Geometry: final body of the model. Coordinates: model frame, mm. Give positions to 0.01 mm unless a question says otherwise; leave off trailing zeros. Write each loop counter-clockwise with the first axis right and the second up, starting at its lowest first coordinate (ties: lowest second). Pieces come first, ordered by that corner, then holes.
Q1. Section B-B (x = 0). Return the cut outline in (y, z), plus the area to 3 significant figures.
Q2. Section D-D (y = -42). Return the cut outline in (x, z), plus the area to 3 significant figures.
Q3. Pin query (flat end, axial travel): pin 1 Ø1 at (y, z) = (-44, -9.5) entering from +X; pin 2 Ø8 at (x, y) = (-6.5, -110) entering from +Z; pin 3 Ø10 at (x, y) = (-4, -24) entering from -Z; pin 4 Ø10 at (x, y) = (8.5, -47) entering from -Z. Return the tip coordinate at first contact, or that it passes through.
Q4. Section C-C (y = -130). Return the cut outline in (x, z).
Q5. Mould query, pull axis Z, two halves, no side actions, for faces 1 (the cylindrical face through (-1.73, -68.53, -7.81)), 2 (the cylindrical face through (-0.113, -127.615, 0.751)), 3 (the flat face through (2, 0, -8)). Classes: +Z half, -Z half, draft (parallel to the pull), parting line (faces both ways), or undercut.
Q6. Line query: line 1 (Z direction, x = 0.5, y = -130); line 2 (Y direction, x = -3.25, z = 0); line 3 (Z direction, x = -4.5, y = -130). Output: solid intervals per line, ascending.
Q7. Section A-A (z = 0). Return the cut outline in (x, y), plus the area to 3 significant figures.
from build123d import *

# Parameters (mm, degrees)
F0_R     = 8
F1_DEPTH = 140
F0_R_2   = 12
F2_DEPTH = 5
F3_SIZE  = 1
F5_R     = 2.5
F6_DEPTH = 20.001


with BuildPart() as f1:
    # F0 (on Front) → F1 (new body)
    with BuildSketch(Plane.XZ):
        Circle(F0_R)
    extrude(amount=F1_DEPTH)

    # F0 (on Front) → F2 (join)
    with BuildSketch(Plane.XZ):
        Circle(F0_R_2)
        Circle(F0_R, mode=Mode.SUBTRACT)
        Circle(F0_R)
    extrude(amount=-F2_DEPTH)

    # F3
    f3_edges = [f1.edges().sort_by_distance(p)[0] for p in [
        (-12, 5, 0),
        (-8, -140, 0),
    ]]
    chamfer(f3_edges, length=F3_SIZE)

    # F5 (on offset) → F6 (cut, through all)
    with BuildSketch(Plane.YZ.offset(-8)):
        with Locations((-130, 0)):
            Circle(F5_R)
    extrude(amount=F6_DEPTH, mode=Mode.SUBTRACT)


solid = f1.part
Computed:
1. outline: (-140, -7) - (-139, -8) - (0, -8) - (0, -12) - (4, -12) - (5, -11) - (5, 11) - (4, 12) - (0, 12) - (0, 8) - (-139, 8) - (-140, 7) - close; hole circle Ø5 at (-130, 0)
1. area: 2,340 mm2
2. outline: circle Ø16 at (0, 0)
2. area: 201 mm2
3. pin 1: passes through
3. pin 2: stops at z = 7.6
3. pin 3: stops at z = -8
3. pin 4: stops at z = -7.19
4. outline: (-7.6, -2.5) arc R8 ccw to (7.6, -2.5) - close; (-7.6, 2.5) - (7.6, 2.5) arc R8 ccw to start
5. face 1: parting line
5. face 2: undercut
5. face 3: draft
6. line 1: z = -7.98 to -2.5, 2.5 to 7.98
6. line 2: y = -140 to -132.5, -127.5 to 5
6. line 3: z = -6.61 to -2.5, 2.5 to 6.61
7. outline: (-12, 0) - (-8, 0) - (-8, -127.5) - (8, -127.5) - (8, 0) - (12, 0) - (12, 4) - (11, 5) - (-11, 5) - (-12, 4) - close; (-8, -139) - (-7, -140) - (7, -140) - (8, -139) - (8, -132.5) - (-8, -132.5) - close
7. area: 2,280 mm2
